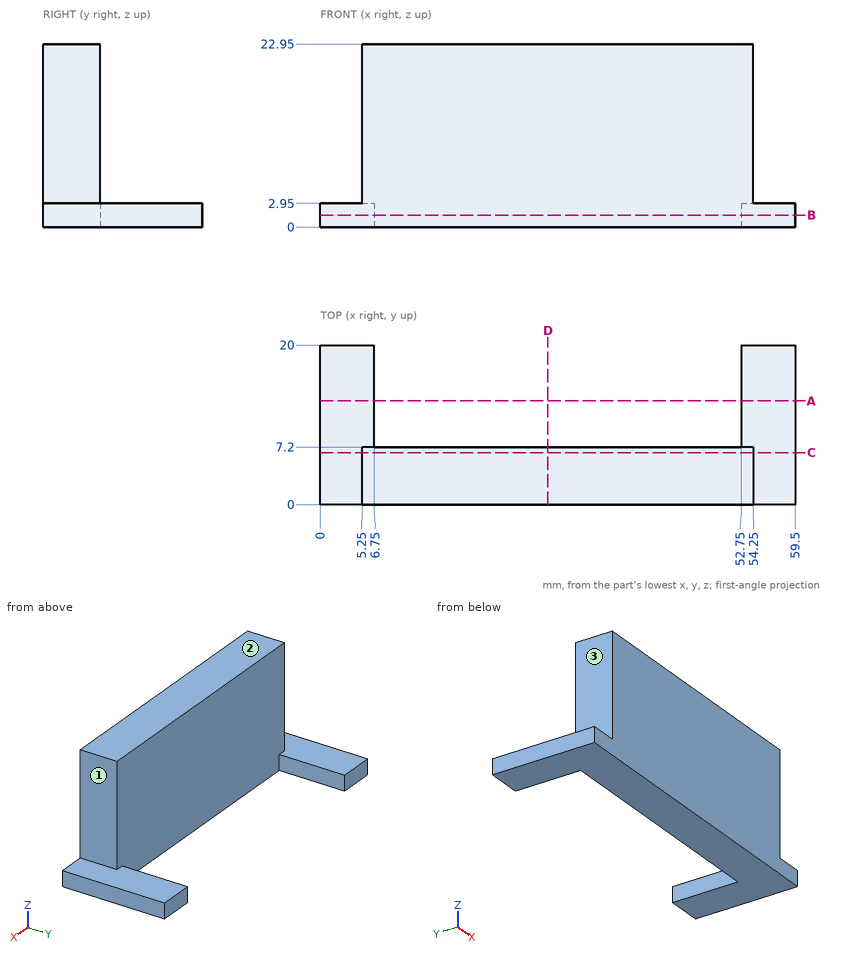
Geometry: see drawing. Coordinates: mm, zero at the bounding-box minimum. A direction names the side the tool comes from. Coordinates: 2 decimals unless noted, no trailing zeros. Write each loop counter-clockwise with the first axis right and the second up, starting at its lowest first coordinate (ties: lowest second). Pieces come first, ordered by that corner, then holes.
1) Section B-B on z = 1.5. Output: boundary loops of the cut face in (x, y).
2) Section C-C on y = 6.5. Output: boundary loops of the cut face in (x, z), and give its area (3 significant figures).
3) Section A-A on y = 13. Output: boundary loops of the cut face in (x, z), and give its area (3 significant figures).
4) Material intervals for line 1 along X through (y, z) = (11, 1); line 2 along Y through (x, z) = (24, 8.5); line 3 along Z through (x, y) = (5, 8.25), sorted ascending.
5) Section D-D on x = 28.5. Output: boundary loops of the cut face in (y, z), and give its area (3 significant figures).
6) Set-up query: the marked faces 1, 2 and 3. Return all of +Z, -Z, +X, -X, +Y, -Y with unobstructed straight access to the full face (end or side cutting, diameter ignored); none if empty.
7) Pin query (flat end, axial travel): pin 1 Ø10 at (y, z) = (8, 8) entering from -X; pin 2 Ø5.5 at (x, y) = (5, 12) entering from +Z; pin 3 Ø1 at (x, z) = (26, 10.5) entering from +Y. Return the tip coordinate at first contact, or that it passes through.
Check result:
1. outline: (0, 0) - (59.5, 0) - (59.5, 20) - (52.75, 20) - (52.75, 7.2) - (6.75, 7.2) - (6.75, 20) - (0, 20) - close
2. outline: (0, 0) - (59.5, 0) - (59.5, 2.95) - (54.25, 2.95) - (54.25, 22.95) - (5.25, 22.95) - (5.25, 2.95) - (0, 2.95) - close
2. area: 1,160 mm2
3. outline: (0, 0) - (6.75, 0) - (6.75, 2.95) - (0, 2.95) - close; (52.75, 0) - (59.5, 0) - (59.5, 2.95) - (52.75, 2.95) - close
3. area: 39.8 mm2
4. line 1: x = 0 to 6.75, 52.75 to 59.5
4. line 2: y = 0 to 7.2
4. line 3: z = 0 to 2.95
5. outline: (0, 0) - (7.2, 0) - (7.2, 22.95) - (0, 22.95) - close
5. area: 165 mm2
6. face 1: +Z, +X, +Y, -Y
6. face 2: +Z, +X, -X, +Y, -Y
6. face 3: +Z, -X, +Y, -Y
7. pin 1: stops at x = 5.25
7. pin 2: stops at z = 2.95
7. pin 3: stops at y = 7.2
